Can you work these out from the model? Positions are in its coordinate system, mm. Round coordinates to 2 decimals unless told otherwise and drop trailing zeros. Loops run counter-clockwise (first coordinate to the right, second up) from the corner with the lowest first, then second, coordinate; pieces in that order, holes last. Notation, with made-up numbers: (-23, 26.5) -> (32, 26.5) arc R26 ccw to (32, 51.5) -> close; hole circle Ø10 at (59, 32.25). An arc over 180 degrees is marked (long way). Use a Markdown table: item, result.
from build123d import *

# Parameters (mm, degrees)
F0_R     = 6.5
F0_R_2   = 3
F1_DEPTH = 5
F2_DEPTH = 5
F3_R     = 1


with BuildPart() as f1:
    # F0 (on Top) → F1 (new body)
    with BuildSketch(Plane.XY):
        Circle(F0_R)
        Circle(F0_R_2, mode=Mode.SUBTRACT)
    extrude(amount=F1_DEPTH)

    # F0 (on Top) → F2 (join)
    with BuildSketch(Plane.XY):
        Circle(F0_R)
        Circle(F0_R_2, mode=Mode.SUBTRACT)
    extrude(amount=F2_DEPTH)

    # F3
    f3_edges = [f1.edges().sort_by_distance(p)[0] for p in [
        (-3, 0, 5),
        (-6.5, 0, 5),
    ]]
    fillet(f3_edges, radius=F3_R)


solid = f1.part
1. I want a section at C-C (z = 2.7). Please give me the cut outline in (x, y).
Answer sheet:
| item | result |
|---|---|
| outline | circle Ø13 at (0, 0); hole circle Ø6 at (0, 0) |
2. Will these pins go through, and if not, where does the flat tip stop? pin 1 Ø2 at (y, z) = (0.5, 1) entering from +X; pin 2 Ø1 at (y, z) = (-2, 1) entering from -X; pin 3 Ø2 at (x, z) = (-5, 1.5) entering from -Y.
Answer sheet:
| item | result |
|---|---|
| pin 1 | stops at x = 6.5 |
| pin 2 | stops at x = -6.32 |
| pin 3 | stops at y = -5.12 |
3. I need wall thicknesses on line 1 (Y direction, x = 0, z = 1.35); line 2 (Y direction, x = -0.75, z = 1.4); line 3 (X direction, y = 1.5, z = 3.05). Which ranges of each line are inside material? Lowest first, please.
Answer sheet:
| item | result |
|---|---|
| line 1 | y = -6.5 to -3, 3 to 6.5 |
| line 2 | y = -6.46 to -2.9, 2.9 to 6.46 |
| line 3 | x = -6.32 to -2.6, 2.6 to 6.32 |
4. I want a section at A-A (y = 0). Please give me the cut outline in (x, z), plus the area to 3 significant figures.
Answer sheet:
| item | result |
|---|---|
| outline | (-6.5, 0) -> (-3, 0) -> (-3, 4) arc R1 ccw to (-4, 5) -> (-5.5, 5) arc R1 ccw to (-6.5, 4) -> close; (3, 0) -> (6.5, 0) -> (6.5, 4) arc R1 ccw to (5.5, 5) -> (4, 5) arc R1 ccw to (3, 4) -> close |
| area | 34.1 mm² |
5. If we mould it in two halves opening along Y, with no side actions, what happens to faces 1 (the cylindrical face through (-5.158, -3.955, 1.972)), 2 (the cylindrical face through (-3, 0, 2)), 3 (the flat face through (-4, -2, 5))? For each: +Y half, -Y half, draft (parallel to the pull), parting line (faces both ways), or undercut.
Answer sheet:
| item | result |
|---|---|
| face 1 | parting line |
| face 2 | undercut |
| face 3 | draft |
